Check sheet for the modelled part. Datum: model origin and axes. Units: mm. A direction names the side the tool comes from. Round coordinates to 2 decimals unless told otherwise and drop trailing zeros. Loops run counter-clockwise (first coordinate to the right, second up) from the corner with the lowest first, then second, coordinate; pieces in that order, holes last. Notation, with made-up numbers: (-27, 12.25) - (26, 12.25) arc R27 ccw to (26, 40.25) - close; hole circle Ø4 at (27.25, 22.5). An arc over 180 degrees is marked (long way). Put each result on its own line as item: value. Start each with the question number.
Item 1: Tool access check on faces 1 (the flat face through (2, -3, -63.017)), 2 (the flat face through (2, 0, -85)), 3 (the flat face through (2, 0, -16)), 4 (the flat face through (2, 121, -81.534)). Record the directions out of +Z, -Z, +X, -X, +Y, -Y that give a thin tool (end or side, any length) a straight path to the whole face; none if there is none.
Item 2: Material ranges on line 1 along Z through (x, y) = (1.8, 99.06); line 2 along Y through (x, z) = (0.1, -14); line 3 along Y through (x, z) = (1.25, -78), recorded low to high.
Item 3: Section check B-B, the plane y = 99.06. Record the cut outline in (x, z) (1 decimal).
Item 4: Gauge pin test, flat ends, axial feed: pin 1 Ø1 at (x, y) = (1, 120.5) entering from +Z; pin 2 Ø1.6 at (x, y) = (1.5, -2) entering from -Z; pin 3 Ø1 at (x, z) = (1.5, -54.5) entering from +Y. Record the tip position at first contact, or that the pin passes through.
Item 5: Draft check along Z on faces 5 (the flat face through (2, -3, -81.509)), 6 (the flat face through (2, 59, 0)), 7 (the flat face through (3.175, 59, -45)), 8 (the flat face through (2, 119.38, -33)). Enter one of: pulls with the +Z half, pulls with the -Z half, needs draft (parallel to the pull), parting line crosses it, or undercut.
Item 6: Section check C-C, the plane y = 20.32. Record the cut outline in (x, z) (3 decimals), and give its area (3 significant figures).
Item 7: Section check A-A, the plane x = 2.45. Give the number of separate pieces and of enclosed holes in the cut face, and give its area (3 significant figures).
from build123d import *

# Parameters (mm, degrees)
BOSS_EXTRUDE1_DEPTH = 3.175
SKETCH2_R           = 1.5875
CUT_EXTRUDE1_DEPTH  = 4.175
SKETCH3_R           = 1.5875
CUT_EXTRUDE2_DEPTH  = 4.175


with BuildPart() as part:
    # Sketch1 → Boss-Extrude1 (new body)
    with BuildSketch(Plane(origin=(0, 0, 0), x_dir=(0, 0, -1), z_dir=(1, 0, 0))):
        Polygon((0, 119.38), (15.621, 119.38), (15.621, 122.555), (28.321, 122.555), (28.321, 119.38), (37.592, 119.38), (37.592, 122.555), (50.292, 122.555), (50.292, 119.38), (59.563, 119.38), (59.563, 122.555), (72.263, 122.555), (72.263, 119.38), (81.534, 119.38), (81.534, 122.555), (87.884, 122.555), (87.884, 0), (81.5086, 0), (81.5086, -6.35), (63.0174, -6.35), (63.0174, 0), (50.2666, 0), (50.2666, -6.35), (31.7754, -6.35), (31.7754, 0), (0, 0), align=None)
    extrude(amount=BOSS_EXTRUDE1_DEPTH)

    # Sketch2 → Cut-Extrude1 (cut, through all)
    with BuildSketch(Plane(origin=(3.175, 0, 0), x_dir=(0, 0, -1), z_dir=(1, 0, 0))):
        with Locations((37.084, 99.06)):
            Circle(SKETCH2_R)
        with Locations((75.184, 99.06)):
            Circle(SKETCH2_R)
    extrude(amount=-CUT_EXTRUDE1_DEPTH, mode=Mode.SUBTRACT)

    # Sketch3 → Cut-Extrude2 (cut, through all)
    with BuildSketch(Plane.ZY):
        with Locations((-81.319973634, 20.32)):
            Circle(SKETCH3_R)
    extrude(amount=-CUT_EXTRUDE2_DEPTH, mode=Mode.SUBTRACT)


solid = part.part
Check result:
1. face 1: +X, -X, -Y
1. face 2: -Z, +X, -X, -Y
1. face 3: +Z, +X, -X, -Y
1. face 4: +X, -X, +Y
2. line 1: -87.88 to -76.77, -73.6 to -38.67, -35.5 to 0
2. line 2: 0 to 119.38
2. line 3: -6.35 to 119.38
3. outline: (0, -87.9) - (3.2, -87.9) - (3.2, -76.8) - (0, -76.8) - close; (0, -73.6) - (3.2, -73.6) - (3.2, -38.7) - (0, -38.7) - close; (0, -35.5) - (3.2, -35.5) - (3.2, 0) - (0, 0) - close
4. pin 1: z = -15.62
4. pin 2: z = -81.51
4. pin 3: y = 119.38
5. face 5: pulls with the -Z half
5. face 6: pulls with the +Z half
5. face 7: needs draft
5. face 8: undercut
6. outline: (0, -87.884) - (3.175, -87.884) - (3.175, -82.907) - (0, -82.907) - close; (0, -79.732) - (3.175, -79.732) - (3.175, 0) - (0, 0) - close
6. area: 269 mm²
7. separate pieces: 1
7. enclosed holes: 3
7. area: 10,800 mm²
